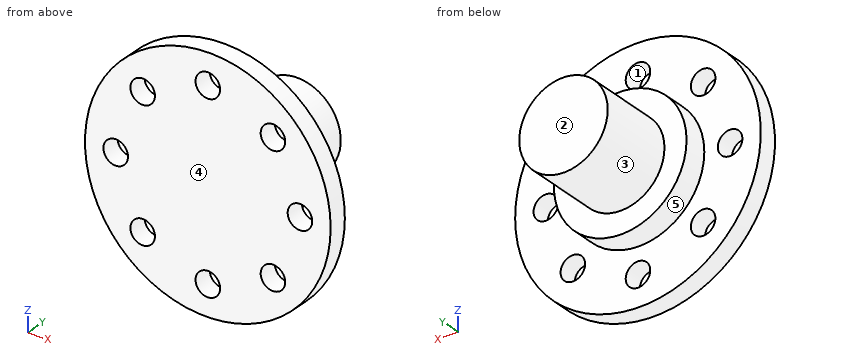
```python
from build123d import *

# Parameters (mm, degrees)
F0_R     = 50
F0_R_2   = 5
F1_DEPTH = 8
F2_R     = 27
F3_DEPTH = 10
F4_R     = 18
F5_DEPTH = 32


with BuildPart() as f1:
    # F0 (on Front) → F1 (new body)
    with BuildSketch(Plane.XZ):
        Circle(F0_R)
        with Locations((-26.516504, -26.516504)):
            Circle(F0_R_2, mode=Mode.SUBTRACT)
        with Locations((0, -37.5)):
            Circle(F0_R_2, mode=Mode.SUBTRACT)
        with Locations((26.516504, -26.516504)):
            Circle(F0_R_2, mode=Mode.SUBTRACT)
        with Locations((-37.5, 0)):
            Circle(F0_R_2, mode=Mode.SUBTRACT)
        with Locations((-26.516504, 26.516504)):
            Circle(F0_R_2, mode=Mode.SUBTRACT)
        with Locations((37.5, 0)):
            Circle(F0_R_2, mode=Mode.SUBTRACT)
        with Locations((0, 37.5)):
            Circle(F0_R_2, mode=Mode.SUBTRACT)
        with Locations((26.516504, 26.516504)):
            Circle(F0_R_2, mode=Mode.SUBTRACT)
    extrude(amount=F1_DEPTH)

    # F2 (on face) → F3 (join)
    with BuildSketch(Plane(origin=(0, 0, 0), x_dir=(-1, 0, 0), z_dir=(0, 1, 0))):
        Circle(F2_R)
    extrude(amount=F3_DEPTH)

    # F4 (on face) → F5 (join)
    with BuildSketch(Plane(origin=(0, 10, 0), x_dir=(-1, 0, 0), z_dir=(0, 1, 0))):
        Circle(F4_R)
    extrude(amount=F5_DEPTH)


solid = f1.part
```
Geometry check sheet. Reference: the model listing, model coordinates, mm. Face numbers are marked on the shaded views. A direction names the side the tool comes from. Give positions to 0.01 mm unless a question says otherwise; leave off trailing zeros. Order: outer loops, then holes, each group sorted by start corner. A loop starts at its lowest first (then second) coordinate and runs counter-clockwise, first axis right, second up. Notation, with made-up numbers: (52.5, 63) - (96.5, 63) arc R29 ccw to (96.5, 95) - close; hole circle Ø9 at (-19.5, 11). An arc over 180 degrees is marked (long way). Write item = value, one per line. Start each with the question number.
1) Scan lines: L1, parallel to Z at x = 0, y = -4; L2, parallel to Z at x = 30, y = -2; L3, parallel to Y at x = 31.5, z = 30.5. Record each from-to range of solid material in increasing order.
2) Section check D-D (z = -10). Enter the section's corners in (x, y).
3) Draft check along Z on the marked faces 1, 2 and 3. Enter one of: released by +Z, released by -Z, zero draft, split by the parting line, or undercut.
4) Section check B-B (x = -37.5). Enter the section's corners in (y, z).
5) Access from +Z, -Z, +X, -X, +Y, -Y to the whole of each face (thin tool, end or side, straight path). Record for the marked faces 4 and 5.
6) Section check C-C (z = -37.5). Enter the section's corners in (x, y).
7) Section check A-A (x = 0). Enter the section's corners in (y, z), then the cut area to 3 significant figures.
8) Gauge pin test, flat ends, axial feed: pin 1 Ø10 at (y, z) = (5.5, 10.5) entering from -X; pin 2 Ø5 at (y, z) = (37, 3) entering from -X; pin 3 Ø16 at (x, z) = (37.5, 0) entering from +Y. Record the tip position at first contact, or that the pin passes through.
Geometry check:
q1.L1 = -50 to -42.5, -32.5 to 32.5, 42.5 to 50
q1.L2 = -40 to -30.1, -22.93 to 22.93, 30.1 to 40
q1.L3 = -8 to 0
q2.outline = (-48.99, -8) - (48.99, -8) - (48.99, 0) - (25.08, 0) - (25.08, 10) - (14.97, 10) - (14.97, 42) - (-14.97, 42) - (-14.97, 10) - (-25.08, 10) - (-25.08, 0) - (-48.99, 0) - close
q3.face_1 = undercut
q3.face_2 = zero draft
q3.face_3 = split by the parting line
q4.outline = (-8, -33.07) - (0, -33.07) - (0, -5) - (-8, -5) - close; (-8, 5) - (0, 5) - (0, 33.07) - (-8, 33.07) - close
q5.face_4 = +Z, -Z, +X, -X, -Y
q5.face_5 = +Y
q6.outline = (-33.07, -8) - (-5, -8) - (-5, 0) - (-33.07, 0) - close; (5, -8) - (33.07, -8) - (33.07, 0) - (5, 0) - close
q7.outline = (-8, -50) - (0, -50) - (0, -42.5) - (-8, -42.5) - close; (-8, -32.5) - (0, -32.5) - (0, -27) - (10, -27) - (10, -18) - (42, -18) - (42, 18) - (10, 18) - (10, 27) - (0, 27) - (0, 32.5) - (-8, 32.5) - close; (-8, 42.5) - (0, 42.5) - (0, 50) - (-8, 50) - close
q7.area = 2,330 mm2
q8.pin_1 = -26.43
q8.pin_2 = -17.99
q8.pin_3 = 0
